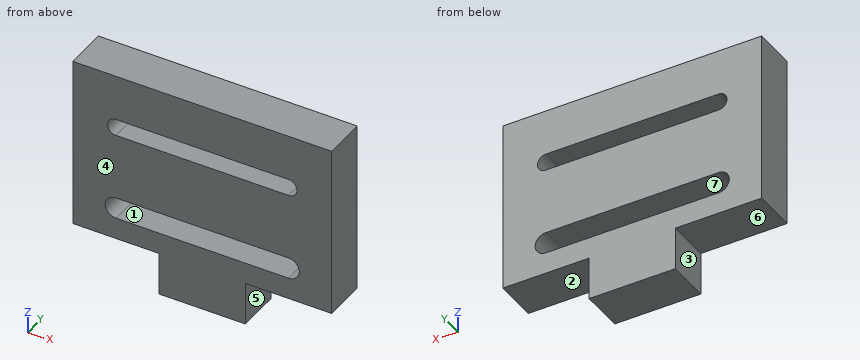
```python
from build123d import *

# Parameters (mm, degrees)
SKETCH1_W           = 38.1
SKETCH1_H           = 6.35
BOSS_EXTRUDE1_DEPTH = 25.4
SKETCH2_W           = 25.4
SKETCH2_H           = 2.5
CUT_EXTRUDE1_DEPTH  = 33.378773911
SKETCH3_W           = 12.7
SKETCH3_H           = 6.35
BOSS_EXTRUDE4_DEPTH = 6.35
SKETCH4_W           = 12.7
SKETCH4_H           = 3.175
CUT_EXTRUDE2_DEPTH  = 10


with BuildPart() as part:
    # Sketch1 → Boss-Extrude1 (new body)
    with BuildSketch(Plane.XY):
        with Locations((0, -9.523336827)):
            Rectangle(SKETCH1_W, SKETCH1_H)
    extrude(amount=BOSS_EXTRUDE1_DEPTH)

    # Sketch2 → Cut-Extrude1 (cut, through all)
    with BuildSketch(Plane(origin=(0, -6.348336827, 0), x_dir=(1, 0, 0), z_dir=(0, 1, 0))):
        with Locations((0, -17.399)):
            Rectangle(SKETCH2_W, SKETCH2_H)
        with BuildLine():
            Line((12.7, -18.649), (12.7, -16.149))
            ThreePointArc((12.7, -16.149), (13.95, -17.399), (12.7, -18.649))
        make_face()
        with BuildLine():
            ThreePointArc((-12.7, -18.649), (-13.95, -17.399), (-12.7, -16.149))
            Line((-12.7, -16.149), (-12.7, -18.649))
        make_face()
    extrude(amount=-CUT_EXTRUDE1_DEPTH, mode=Mode.SUBTRACT)

    # Sketch3 → Boss-Extrude4 (add)
    with BuildSketch(Plane(origin=(0, 0, 0), x_dir=(-1, 0, 0), z_dir=(0, 0, -1))):
        with Locations((0, -9.523336827)):
            Rectangle(SKETCH3_W, SKETCH3_H)
    extrude(amount=BOSS_EXTRUDE4_DEPTH)

    # Sketch4 → Cut-Extrude2 (cut)
    with BuildSketch(Plane(origin=(0, -6.348336827, 0), x_dir=(1, 0, 0), z_dir=(0, 1, 0))):
        with Locations((-6.35, -4.7625)):
            Rectangle(SKETCH4_W, SKETCH4_H)
        with BuildLine():
            ThreePointArc((-12.7, -6.35), (-14.2875, -4.7625), (-12.7, -3.175))
            Line((-12.7, -3.175), (-12.7, -6.35))
        make_face()
        with Locations((6.35, -4.7625)):
            Rectangle(SKETCH4_W, SKETCH4_H)
        with BuildLine():
            Line((12.7, -6.35), (12.7, -3.175))
            ThreePointArc((12.7, -3.175), (14.2875, -4.7625), (12.7, -6.35))
        make_face()
    extrude(amount=-CUT_EXTRUDE2_DEPTH, mode=Mode.SUBTRACT)


solid = part.part
```
Geometry: final body of the model. Coordinates: model frame, mm. Face numbers are marked on the shaded views. A direction names the side the tool comes from. Round coordinates to 2 decimals unless told otherwise and drop trailing zeros. Order: outer loops, then holes, each group sorted by start corner. A loop starts at its lowest first (then second) coordinate and runs counter-clockwise, first axis right, second up. Notation, with made-up numbers: (-23, 5.5) -> (4, 5.5) arc R22 ccw to (4, 26.5) -> close; hole circle Ø6 at (63, 23.25). An arc over 180 degrees is marked (long way). Write each question's results on one line, items separated by ' | '.
Q1. Section query A-A (x = 10.5). Output: boundary loops of the cut face in (y, z) (3 decimals), and give its area (3 significant figures).
Response values:
outline: (-12.698, 0) -> (-6.348, 0) -> (-6.348, 3.175) -> (-12.698, 3.175) -> close; (-12.698, 6.35) -> (-6.348, 6.35) -> (-6.348, 16.149) -> (-12.698, 16.149) -> close; (-12.698, 18.649) -> (-6.348, 18.649) -> (-6.348, 25.4) -> (-12.698, 25.4) -> close | area: 125 mm²
Q2. Section query D-D (x = -5.5). Output: boundary loops of the cut face in (y, z) (3 decimals).
Response values:
outline: (-12.698, -6.35) -> (-6.348, -6.35) -> (-6.348, 3.175) -> (-12.698, 3.175) -> close; (-12.698, 6.35) -> (-6.348, 6.35) -> (-6.348, 16.149) -> (-12.698, 16.149) -> close; (-12.698, 18.649) -> (-6.348, 18.649) -> (-6.348, 25.4) -> (-12.698, 25.4) -> close
Q3. Pin query (flat end, axial travel): pin 1 Ø1 at (x, y) = (11, -7) entering from -Z; pin 2 Ø3 at (y, z) = (-9.5, -2.5) entering from -X. Return the tip coordinate at first contact, or that it passes through.
Response values:
pin 1: z = 0 | pin 2: x = -6.35
Q4. Section query B-B (z = 4.5). Output: boundary loops of the cut face in (x, y), and give its area (3 significant figures).
Response values:
outline: (-19.05, -12.7) -> (-14.27, -12.7) -> (-14.27, -6.35) -> (-19.05, -6.35) -> close; (14.27, -12.7) -> (19.05, -12.7) -> (19.05, -6.35) -> (14.27, -6.35) -> close | area: 60.8 mm²
Q5. Access query for the marked faces 4, 5, 6 and 7. Directions: +Z, -Z, +X, -X, +Y, -Y. A direction counts if a zero-diameter tool reaches every point of the face in a straight line with its end or side. Return the directions, or none.
Response values:
face 4: +Z, -Z, +X, -X, -Y | face 5: -Z, +X, +Y, -Y | face 6: -Z, -X, +Y, -Y | face 7: +Y, -Y
Q6. Section query C-C (y = -9.25). Count the separate pieces of the cut face and the enclosed holes in it, and give its area (3 significant figures).
Response values:
separate pieces: 1 | enclosed holes: 2 | area: 891 mm²
Q7. Ray query, line 1 along Z through (x, y) = (-10, -8) (3 decimals); line 2 along Z through (x, y) = (-4, -7) (3 decimals); line 3 along X through (y, z) = (-10, -0.5). Return the intervals inside material, ascending.
Response values:
line 1: 0 to 3.175, 6.35 to 16.149, 18.649 to 25.4 | line 2: -6.35 to 3.175, 6.35 to 16.149, 18.649 to 25.4 | line 3: -6.35 to 6.35
Q8. Pull-direction query (Z, two-part tool) for the marked faces 1, 2 and 3; classes: released by +Z, released by -Z, zero draft, split by the parting line, or undercut.
Response values:
face 1: undercut | face 2: released by -Z | face 3: zero draft
